Could you check a few things on this model? Use its own coordinates, in mm. Give positions to 0.01 mm unless a question says otherwise; leave off trailing zeros. Order: outer loops, then holes, each group sorted by start corner. A loop starts at its lowest first (then second) coordinate and runs counter-clockwise, first axis right, second up. Notation, with made-up numbers: (50, 53.5) - (61, 53.5) arc R22 cw to (61, 79.5) - close; hole circle Ø11 at (-30.5, 5). An arc over 180 degrees is marked (long way). Put each result on its own line as item: value.
from build123d import *

# Parameters (mm, degrees)
SKETCH1_W           = 330
SKETCH1_H           = 230
BOSS_EXTRUDE1_DEPTH = 2
CUT_EXTRUDE1_DEPTH  = 2
FILLET1_R           = 30


with BuildPart() as part:
    # Sketch1 → Boss-Extrude1 (new body)
    with BuildSketch(Plane.XY):
        Rectangle(SKETCH1_W, SKETCH1_H)
    extrude(amount=BOSS_EXTRUDE1_DEPTH)

    # Sketch2 → Cut-Extrude1 (cut)
    with BuildSketch(Plane(origin=(0, 0, 0), x_dir=(-1, 0, 0), z_dir=(0, 0, -1))):
        with BuildLine():
            Line((-140, 75), (-66, 75))
            ThreePointArc((-66, 75), (-62.464466094, 73.535533906), (-61, 70))
            Line((-61, 70), (-61, -44))
            ThreePointArc((-61, -44), (-62.464466094, -47.535533906), (-66, -49))
            Line((-66, -49), (-140, -49))
            ThreePointArc((-140, -49), (-143.535533906, -47.535533906), (-145, -44))
            Line((-145, -44), (-145, 70))
            ThreePointArc((-145, 70), (-143.535533906, 73.535533906), (-140, 75))
        make_face()
    extrude(amount=-CUT_EXTRUDE1_DEPTH, mode=Mode.SUBTRACT)

    # Fillet1
    fillet1_edges = [part.edges().sort_by_distance(p)[0] for p in [
        (165, -115, 1),
        (-165, -115, 1),
        (-165, 115, 1),
        (165, 115, 1),
    ]]
    fillet(fillet1_edges, radius=FILLET1_R)


solid = part.part
1) If I drill on line 1 (X direction, y = 50, z = 1.35); line 2 (X direction, y = -48, z = 1.3); line 3 (X direction, y = 100.5, z = 0.4), over which ranges is the centre line in solid material (lowest first)? Write a range as [from, to].
Filled in:
line 1: x = [-165, 61], [145, 165]
line 2: x = [-165, 63], [143, 165]
line 3: x = [-160.69, 160.69]
2) Suppose I cut it at A-A, the plane y = 61.5. List the corners of the cut face in (x, z) for me.
Filled in:
outline: (-165, 0) - (61, 0) - (61, 2) - (-165, 2) - close; (145, 0) - (165, 0) - (165, 2) - (145, 2) - close
3) We'd pull the mould along X, two halves only. Please class faces 1 (the cylindrical face through (155.979, 106.445, 1.014)), 2 (the flat face through (-39, 2, 2)), 3 (the cylindrical face through (-156.445, 105.979, 1.014)): pulls with the +X half, pulls with the -X half, needs draft (parallel to the pull), parting line crosses it, or undercut.
Filled in:
face 1: pulls with the +X half
face 2: needs draft
face 3: pulls with the -X half
4) Suppose I cut it at B-B, the plane z = 1.7. List the corners of the cut face in (x, y) for me, and give its area (3 significant figures).
Filled in:
outline: (-165, -85) arc R30 ccw to (-135, -115) - (135, -115) arc R30 ccw to (165, -85) - (165, 85) arc R30 ccw to (135, 115) - (-135, 115) arc R30 ccw to (-165, 85) - close; hole (61, -44) arc R5 ccw to (66, -49) - (140, -49) arc R5 ccw to (145, -44) - (145, 70) arc R5 ccw to (140, 75) - (66, 75) arc R5 ccw to (61, 70) - close
area: 64,700 mm^2
